Autodesk Inventor part; units mm, degrees
ref_plane "Work Plane1" through (0, 145, 0) normal (0, 1, 0) x (-1, 0, 0)
ref_plane "YZ Plane" through (0, 0, 0) normal (1, 0, 0) x (0, 1, 0)
ref_plane "XY Plane" through (0, 0, 0) normal (0, 0, 1) x (1, 0, 0)
sketch "Sketch2" plane through (0, 0, 0) normal (0, 0, 1) x (1, 0, 0)
  circle A0 centre (0, 0) radius 61
  circle A1 centre (0, 0) radius 28
  line L0 (0, 68.8089) -> (0, -61.0943)
  line L1 (-74.2561, 0) -> (92.1735, 0)
  circle A2 centre (0, 50) radius 3.665
  circle A3 centre (-25, 43.3013) radius 3.665
  circle A4 centre (-43.3013, 25) radius 3.665
  circle A5 centre (-50, 0) radius 3.665
  circle A6 centre (-43.3013, -25) radius 3.665
  circle A7 centre (-25, -43.3013) radius 3.665
  circle A8 centre (0, -50) radius 3.665
  circle A9 centre (25, -43.3013) radius 3.665
  circle A10 centre (43.3013, -25) radius 3.665
  circle A11 centre (50, 0) radius 3.665
  circle A12 centre (43.3013, 25) radius 3.665
  circle A13 centre (25, 43.3013) radius 3.665
  dimension "d0" = 122
  dimension "d1" = 56
  dimension "d2" = 7.33
  dimension "d4" = 50
  dimension "d7" = 360
extrude "Extrusion1" add sketch "Sketch2" along normal blind 11 contours L1 A11 A1 L0 A2 A0 | A0 L0 A8 A1 L1 A11 | L0 A2 A1 L1 A5 A0 | A0 L1 A5 A1 L0 A8
ref_plane "Work Plane1" through (0, 145, 0) normal (0, 1, 0) x (-1, 0, 0)
sketch "Sketch4" plane through (0, 0, 0) normal (0, 0, -1) x (-1, 0, 0)
  circle A0 centre (0, 0) radius 28
  circle A1 centre (0, 0) radius 33.5
  line L0 (-79.8111, 140.7115) -> (80.5184, 140.7115) construction
  dimension "d12" = 56
  dimension "d13" = 67
revolve "Revolution1" add sketch "Sketch4" angle 38 about axis through (79.8111, 140.7115, 0) along (-1, 0, 0)
sketch "Sketch5" plane through (0, 29.8293, 86.6306) normal (0, 0.6157, 0.788) x (1, 0, 0)
  circle A0 centre (0, 0) radius 61
  circle A1 centre (0, 0) radius 28
  line L0 (25.8703, 42.9334) -> (25.8703, -86.9698)
  line L1 (-48.3858, -25.8755) -> (118.0439, -25.8755)
  circle A2 centre (25.8703, 42.787) radius 3.665
  circle A3 centre (1.0109, 49.9898) radius 3.665
  circle A4 centre (-24.1194, 43.7979) radius 3.665
  circle A5 centre (-42.787, 25.8703) radius 3.665
  circle A6 centre (-49.9898, 1.0109) radius 3.665
  circle A7 centre (-43.7979, -24.1194) radius 3.665
  circle A8 centre (-25.8703, -42.787) radius 3.665
  circle A9 centre (-1.0109, -49.9898) radius 3.665
  circle A10 centre (24.1194, -43.7979) radius 3.665
  circle A11 centre (42.787, -25.8703) radius 3.665
  circle A12 centre (49.9898, -1.0109) radius 3.665
  circle A13 centre (43.7979, 24.1194) radius 3.665
  point P0 (0, 29.8293)
  dimension "d17" = 122
  dimension "d18" = 56
  dimension "d19" = 7.33
  dimension "d20" = 50
  dimension "d21" = 360
extrude "Extrusion2" add sketch "Sketch5" along normal blind 11 contours L1 A1 L0 | A0 L1 A11 L0 A10 | L0 A10 L1 A11 A0 picked at (22.9817, -20.4121)
properties part number "crazy"
Input: part model. Units: mm. Frame: model coordinates. A direction names the side the tool comes from. Give positions to 0.01 mm unless a question says otherwise; leave off trailing zeros. Order: outer loops, then holes, each group sorted by start corner. A loop starts at its lowest first (then second) coordinate and runs counter-clockwise, first axis right, second up. Notation, with made-up numbers: (-12.5, -3.75) - (44.5, -3.75) arc R16 cw to (44.5, 2.25) - close; hole circle Ø8 at (-32, -32.5). An arc over 180 degrees is marked (long way). Answer as a JSON object with one key per item and string values. Group by question number.
Q1. First-contact query: pin 1 Ø2 at (x, y) = (11.5, -12) entering from +Z; pin 2 Ø6 at (x, y) = (-50, 0) entering from -Z; pin 3 Ø8 at (x, z) = (-10, 26) entering from -Y. Flat tips, straight axial feed; report the tip coordinate or a pass-through.
Q2. Cut plane A-A, the plane x = 50. Output: boundary loops of the cut face in (y, z) (3 decimals).
Q3. Cut plane B-B, the plane y = -50. Output: boundary loops of the cut face in (x, z) (3 decimals).
Q4. Line query: probe 1 along Y at (x, z) = (20, 68); probe 2 along Y at (x, z) = (-11, 53.5); probe 3 along Y at (x, z) = (0, 5) (3 decimals). Output: solid intervals per line, ascending.
Q5. Mould query, pull axis Y, two halves, no side actions, for faces 1 (the face through (29.366, 66.017, 65.239)), 2 (the face through (-48.408, 62.417, 68.052)), 3 (the face through (53.375, 33.478, 90.662)). Classes: pulls with the +Y half, pulls with the -Y half, needs draft (parallel to the pull), parting line crosses it, or undercut.
Q6. Set-up query: faces 4 (the face through (-46, -27.48, 5.42)), 5 (the face through (1.9, 28.1, 11)), 6 (the face through (47.09, 2.23, 5.42)). Return all of +Z, -Z, +X, -X, +Y, -Y with unobstructed straight access to the full face (end or side cutting, diameter ignored); none if empty.
Q7. Cut plane C-C, the plane x = 0. Count the separate pieces of the cut face and the enclosed holes in it, then the cut area to 3 significant figures.
Results:
{
 "1": {"pin 1": "z = 131.71", "pin 2": "z = 107.59", "pin 3": "y = -31.19"},
 "2": {"outline": "(-34.943, 0) - (-3.665, 0) - (-3.665, 11) - (-34.943, 11) - close; (2.294, 108.144) - (26.145, 89.509) - (32.917, 98.177) - (9.066, 116.812) - close; (3.665, 0) - (34.943, 0) - (34.943, 11) - (3.665, 11) - close; (31.921, 84.997) - (57.365, 65.118) - (64.137, 73.786) - (38.693, 93.665) - close"},
 "3": {"outline": "(-34.943, 0) - (-3.665, 0) - (-3.665, 11) - (-34.943, 11) - close; (3.665, 0) - (34.943, 0) - (34.943, 11) - (3.665, 11) - close"},
 "4": {"probe 1": "-12.46 to -4.46, 40.49 to 49.42, 53.68 to 71.54", "probe 2": "-23.13 to -16.92, 38.96 to 45.67, 72.23 to 80.09", "probe 3": "-61 to -53.665, -46.335 to -27.926, 28 to 46.335, 53.665 to 61"},
 "5": {"face 1": "undercut", "face 2": "parting line crosses it", "face 3": "undercut"},
 "6": {"face 4": "+Z, -Z", "face 5": "none", "face 6": "-Z"},
 "7": {"separate pieces": "6", "enclosed holes": "0", "area": "2,040 mm^2"}
}
